Geometry check sheet. Reference: drawing and pictorial views, mm from the part's lowest x, y, z. A direction names the side the tool comes from. Give positions to 0.01 mm unless a question says otherwise; leave off trailing zeros. Write each loop counter-clockwise with the first axis right and the second up, starting at its lowest first coordinate (ties: lowest second). Pieces come first, ordered by that corner, then holes. Notation, with made-up numbers: (-32.75, -23) - (-1.75, -23) arc R14 cw to (-1.75, -2) - close; hole circle Ø7 at (-19, 10.5). An arc over 180 degrees is marked (long way). Write item = value, one per line. Start each with the question number.
(1) Depth check by flat-ended pin: pin 1 Ø2.5 at (y, z) = (3.5, 27) entering from -X; pin 2 Ø3.5 at (x, y) = (17, 7) entering from -Z; pin 3 Ø3.5 at (y, z) = (2.5, 26.5) entering from +X; pin 4 Ø2.5 at (x, z) = (16.3, 12.5) entering from +Y. Enter the tip coordinate at first touch or a pass-through.
(2) Section check B-B, the plane z = 26. Enter the section's corners in (x, y).
(3) Access from +Z, -Z, +X, -X, +Y, -Y to the whole of each face (thin tool, end or side, straight path). Record for the marked faces 1 and 2.
(4) Section check A-A, the plane x = 38.8. Enter the section's corners in (y, z), plus the area to 3 significant figures.
(5) Section check D-D, the plane x = 25. Enter the section's corners in (y, z), plus the area to 3 significant figures.
(6) Section check C-C, the plane y = 8. Enter the section's corners in (x, z).
(7) Thickness scan on L1, parallel to Z at x = 16.3, y = 13; L2, parallel to Y at x = 36, z = 26.4; L3, parallel to Y at x = 39, z = 7. Record the ranges inside material, lowest first.
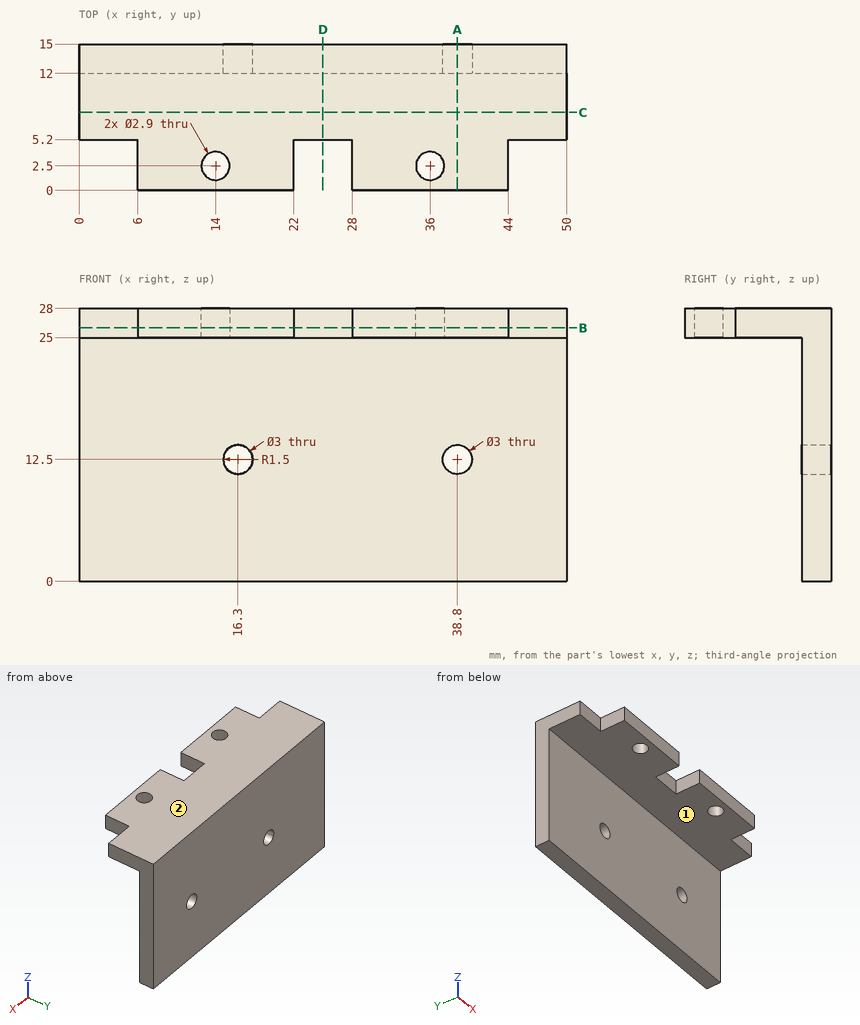
Model answer:
q1.pin_1 = 6
q1.pin_2 = 25
q1.pin_3 = 44
q1.pin_4 = through
q2.outline = (0, 5.2) - (6, 5.2) - (6, 0) - (22, 0) - (22, 5.2) - (28, 5.2) - (28, 0) - (44, 0) - (44, 5.2) - (50, 5.2) - (50, 15) - (0, 15) - close; hole circle Ø2.9 at (14, 2.5); hole circle Ø2.9 at (36, 2.5)
q3.face_1 = -Z, +X, -X, -Y
q3.face_2 = +Z, +X, -X, +Y, -Y
q4.outline = (0, 25) - (12, 25) - (12, 14) - (15, 14) - (15, 28) - (0, 28) - close; (12, 0) - (15, 0) - (15, 11) - (12, 11) - close
q4.area = 111 mm²
q5.outline = (5.2, 25) - (12, 25) - (12, 0) - (15, 0) - (15, 28) - (5.2, 28) - close
q5.area = 104 mm²
q6.outline = (0, 25) - (50, 25) - (50, 28) - (0, 28) - close
q7.L1 = 0 to 11, 14 to 28
q7.L2 = 0 to 1.05, 3.95 to 15
q7.L3 = 12 to 15
